The listing builds one solid part. Answer for the finished solid, in the listing's coordinates (mm). Coordinates: 2 decimals unless noted, no trailing zeros. Loops run counter-clockwise (first coordinate to the right, second up) from the corner with the lowest first, then second, coordinate; pieces in that order, holes last. Notation, with made-up numbers: (-19.5, 61) - (-4.5, 61) arc R16 ccw to (-4.5, 80) - close; hole circle Ø6 at (-29.5, -19.75). An arc over 180 degrees is marked (long way). One line per question, with ' | ' between items.
from build123d import *

# Parameters (mm, degrees)
SKETCH_1_R      = 4
SKETCH_1_R_2    = 0.5
EXTRUDE_1_DEPTH = 5


with BuildPart() as part:
    # 草圖1 → 填料-伸長1 (new body)
    with BuildSketch(Plane.XY):
        with BuildLine():
            ThreePointArc((-16.161165235, 8.838834765), (-37.5, 0), (-16.161165235, -8.838834765))
            ThreePointArc((-16.161165235, -8.838834765), (-15.608913833, -8.304841047), (-15.039028639, -7.789708279))
            ThreePointArc((-15.039028639, -7.789708279), (-9.525276207, -5.376821949), (-3.625257572, -6.56563078))
            ThreePointArc((-3.625257572, -6.56563078), (0, -7.5), (3.625257572, -6.56563078))
            ThreePointArc((3.625257572, -6.56563078), (9.525276207, -5.376821949), (15.039028639, -7.789708279))
            ThreePointArc((15.039028639, -7.789708279), (15.608913833, -8.304841047), (16.161165235, -8.838834765))
            ThreePointArc((16.161165235, -8.838834765), (37.5, 0), (16.161165235, 8.838834765))
            ThreePointArc((16.161165235, 8.838834765), (15.608913833, 8.304841047), (15.039028639, 7.789708279))
            ThreePointArc((15.039028639, 7.789708279), (9.525276207, 5.376821949), (3.625257572, 6.56563078))
            ThreePointArc((3.625257572, 6.56563078), (0, 7.5), (-3.625257572, 6.56563078))
            ThreePointArc((-3.625257572, 6.56563078), (-9.525276207, 5.376821949), (-15.039028639, 7.789708279))
            ThreePointArc((-15.039028639, 7.789708279), (-15.608913833, 8.304841047), (-16.161165235, 8.838834765))
        make_face()
        with Locations((-25, 0)):
            Circle(SKETCH_1_R, mode=Mode.SUBTRACT)
        with Locations((25, 0)):
            Circle(SKETCH_1_R, mode=Mode.SUBTRACT)
        with Locations((-10, 0)):
            Circle(SKETCH_1_R_2, mode=Mode.SUBTRACT)
        with Locations((10, 0)):
            Circle(SKETCH_1_R_2, mode=Mode.SUBTRACT)
    extrude(amount=EXTRUDE_1_DEPTH)


solid = part.part
Item 1: The mould has two halves that part along Y. Classify faces 1 (the face through (9.44, -5.37, 2.46)), 2 (the face through (-1, 0, 0)), 3 (the face through (21.8, -2.4, 2.5)), 4 (the face through (37.493, -0.412, 2.465)): pulls with the +Y half, pulls with the -Y half, needs draft (parallel to the pull), parting line crosses it, or undercut.
Taken from the geometry:
face 1: pulls with the -Y half | face 2: needs draft | face 3: undercut | face 4: parting line crosses it
Item 2: Find section B-B, the plane z = 4.1. Write down the section's boundary in (x, y), plus the area to 3 significant figures.
Taken from the geometry:
outline: (-16.16, -8.84) arc R22.86 cw to (-15.04, -7.79) arc R10 cw to (-3.63, -6.57) arc R7.5 ccw to (3.63, -6.57) arc R10 cw to (15.04, -7.79) arc R22.86 cw to (16.16, -8.84) arc R12.5 ccw (long way) to (16.16, 8.84) arc R22.86 cw to (15.04, 7.79) arc R10 cw to (3.63, 6.57) arc R7.5 ccw to (-3.63, 6.57) arc R10 cw to (-15.04, 7.79) arc R22.86 cw to (-16.16, 8.84) arc R12.5 ccw (long way) to start; hole circle Ø8 at (-25, 0); hole circle Ø1 at (-10, 0); hole circle Ø1 at (10, 0); hole circle Ø8 at (25, 0) | area: 1,200 mm2
Item 3: Find section A-A, the plane x = 25. Write down the section's boundary in (y, z), plus the area to 3 significant figures.
Taken from the geometry:
outline: (-12.5, 0) - (-4, 0) - (-4, 5) - (-12.5, 5) - close; (4, 0) - (12.5, 0) - (12.5, 5) - (4, 5) - close | area: 85.0 mm2
Item 4: Find the intervals of material crossed by line 1 (Y direction, x = -25, z = 1.45); line 2 (X direction, y = -1.5, z = 2.35); line 3 (Y direction, x = 23, z = 0.8), in increasing order. Write a range as [from, to].
Taken from the geometry:
line 1: y = [-12.5, -4], [4, 12.5] | line 2: x = [-37.41, -28.71], [-21.29, 21.29], [28.71, 37.41] | line 3: y = [-12.34, -3.46], [3.46, 12.34]
Item 5: Find section D-D, the plane x = -27.5. Write down the section's boundary in (y, z), plus the area to 3 significant figures.
Taken from the geometry:
outline: (-12.25, 0) - (-3.12, 0) - (-3.12, 5) - (-12.25, 5) - close; (3.12, 0) - (12.25, 0) - (12.25, 5) - (3.12, 5) - close | area: 91.2 mm2
Item 6: Each of these flat-tipped pins is pushed along its axis until it touches: pin 1 Ø5 at (x, y) = (-25, 0) entering from -Z; pin 2 Ø1 at (x, z) = (-23, 4.5) entering from -Y; pin 3 Ø3 at (x, z) = (-6.5, 1.5) entering from +Y; pin 4 Ø3 at (x, z) = (17, 1) entering from -Y. Where does it stop, or does it pass through?
Taken from the geometry:
pin 1: passes through | pin 2: stops at y = -12.41 | pin 3: stops at y = 5.94 | pin 4: stops at y = -10.68
Item 7: Find section C-C, the plane y = -1.5. Write down the section's boundary in (x, z).
Taken from the geometry:
outline: (-37.41, 0) - (-28.71, 0) - (-28.71, 5) - (-37.41, 5) - close; (-21.29, 0) - (21.29, 0) - (21.29, 5) - (-21.29, 5) - close; (28.71, 0) - (37.41, 0) - (37.41, 5) - (28.71, 5) - close
